Geometry check sheet. Reference: the model listing, model coordinates, mm. Face numbers are marked on the shaded views. A direction names the side the tool comes from. Give positions to 0.01 mm unless a question says otherwise; leave off trailing zeros. One line per question, with ' | ' between items. Start each with the question number.
Q1. Thickness scan on L1, parallel to Z at x = -89.5, y = -76; L2, parallel to Y at x = 70, z = 10.8; L3, parallel to Z at x = -86, y = -62. Record the ranges inside material, lowest first. Write a range as [from, to].
Q2. Set-up check for the marked faces 1 and 2: record each of +Z, -Z, +X, -X, +Y, -Y from which the full face is reachable in a straight line by a thin tool's end or side.
Q3. Section check A-A on z = 16.5. Count the separate pieces of the cut face and the enclosed holes in it, and give its area (3 significant figures).
Q4. Gauge pin test, flat ends, axial feed: P1, Ø5, axis at x = -50.5, y = 0, coming from the -Z side; P2, Ø2, axis at x = 66, z = 16.5, coming from the -Y side; P3, Ø4, axis at x = -24, z = 17, coming from the +Y side. Record the tip position at first contact, or that the pin passes through.
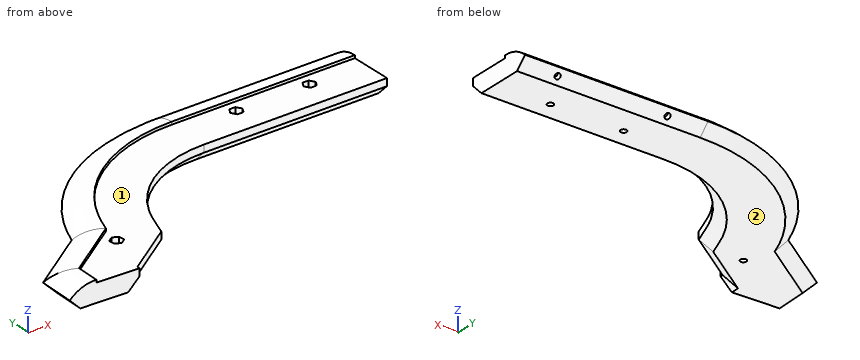
Autodesk Inventor part; units mm, degrees
ref_plane "Work Plane1" through (50, 0, 0) normal (-1, 0, 0) x (0, 0, 1)
ref_plane "Work Plane2" through (0, 14.1421, 14.1421) normal (0, 0, 1) x (1, 0, 0)
ref_plane "YZ Plane" through (0, 0, 0) normal (1, 0, 0) x (0, 1, 0)
sketch "Sketch1" plane through (0, 0, 0) normal (1, 0, 0) x (0, 1, 0)
  circle A0 centre (0, 0) radius 20
  line L0 (8.5, 8.5) -> (-16.9, 8.5)
  line L1 (8.5, 8.5) -> (8.5, -16.9)
  line L2 (0, 0) -> (0, 20)
  line L3 (0, 20) -> (-60.9241, 20)
  line L4 (-60.9241, 20) -> (-60.9241, 18.5)
  line L5 (-60.9241, 18.5) -> (0, 18.5)
  line L6 (0, 18.5) -> (0, 20)
  line L7 (0, 0) -> (14.1421, 14.1421)
  line L8 (0, 0) -> (20, 0)
  line L9 (-16.9, 8.5) -> (-16.9, 18.5)
  line L10 (-16.9, 8.5) -> (-22.9, 14.5)
  line L11 (-22.9, 14.5) -> (-22.9, 18.5)
  line L12 (12.3744, 12.3744) -> (12.1502, 13.2109)
  line L13 (11.3137, 13.435) -> (9.2071, 11.3284)
  line L14 (9.4313, 10.4919) -> (10.2678, 10.2678)
  line L15 (8.5, 8.5) -> (8.5, -16.9)
  line L16 (20, 0) -> (20, -60.9241)
  line L17 (20, -60.9241) -> (18.5, -60.9241)
  line L18 (18.5, -60.9241) -> (18.5, 0)
  line L19 (8.5, -16.9) -> (18.5, -16.9)
  line L20 (8.5, -16.9) -> (14.5, -22.9)
  line L21 (14.5, -22.9) -> (18.5, -22.9)
  arc A1 (9.2071, 11.3284) -> (9.4313, 10.4919) centre (9.5607, 10.9749) ccw
  arc A2 (12.1502, 13.2109) -> (11.3137, 13.435) centre (11.6673, 13.0815) ccw
  line L22 (10.4311, 10.4311) -> (9.483, 10.6851)
  arc A3 (9.3485, 11.187) -> (9.483, 10.6851) centre (9.5607, 10.9749) ccw
  line L23 (9.3485, 11.187) -> (11.4551, 13.2936)
  arc A4 (11.957, 13.1591) -> (11.4551, 13.2936) centre (11.6673, 13.0815) ccw
  line L24 (11.957, 13.1591) -> (12.2111, 12.2111)
  point P0 (0, 8.5)
  point P1 (-17.7041, 9.3041)
  point P2 (-16.9, 10.6953)
  dimension "d0" = 40
  dimension "d1" = 25.4
  dimension "d2" = 1.5
  dimension "d4" = 45
  dimension "d6" = 45
  dimension "d7" = 4
  dimension "d8" = 10
  dimension "d10" = 2.5
  dimension "d11" = 2.5
  dimension "d12" = 60
  dimension "d13" = 1.5
  dimension "d15" = 0.5
  dimension "d16" = 0.2
extrude "Extrusion1" add sketch "Sketch1" along normal blind 100 contours L7 L12 A2 L13 A1 L14 L0 L2 A0 | L7 L24 A4 L23 A3 L22 L14 A1 L13 A2 L12 | L5 L2 L0 L9 A0 | A0 L9 L5 | L7 L22 A3 L23 A4 L24 | L9 L10 A0 | A0 L10 L11 L5 L9
sketch "Sketch2" plane through (0, -22.9, 18.5) normal (0, 0, 1) x (1, 0, 0)
  line L0 (0, 22.9) -> (0, 0)
  line L1 (0, 0) -> (100, 0)
  line L2 (100, 22.9) -> (100, 0)
  line L3 (0, 22.9) -> (100, 22.9)
  line L4 (28.3257, 13.1) -> (26.6514, 16)
  line L5 (26.6514, 16) -> (28.3257, 18.9)
  line L6 (28.3257, 18.9) -> (31.6743, 18.9)
  line L7 (31.6743, 18.9) -> (33.3486, 16)
  line L8 (33.3486, 16) -> (31.6743, 13.1)
  line L9 (31.6743, 13.1) -> (28.3257, 13.1)
  line L10 (0, 6) -> (100, 6)
  circle A0 centre (30, 16) radius 1.65
  dimension "d20" = 10
  dimension "d21" = 5.8
  dimension "d22" = 30
  dimension "d25" = 3.3
extrude "Extrusion2" cut sketch "Sketch2" against normal blind 6 contours L4 L5 L6 L7 L8 L9 | A0
extrude "Extrusion3" cut sketch "Sketch2" against normal through all contours A0
sketch "Sketch3" plane through (0, -22.9, 18.5) normal (0, 0, 1) x (1, 0, 0)
  line L0 (0, 37.0421) -> (100, 37.0421)
  line L1 (0, 0) -> (100, 0)
  line L2 (0, 22.9) -> (0, 0)
  line L3 (0, 22.9) -> (0, 37.0421)
  line L4 (2.4384, 37.0421) -> (17.8575, 0)
  line L5 (0, 0) -> (100, 0)
  line L6 (2.4384, 37.0421) -> (0, 42.9)
  point P0 (0, 26.9698)
  dimension "d28" = 112.6
sketch "Sketch4" plane through (100, 14.1421, 14.1421) normal (0, 0.7071, -0.7071) x (-1, 0, 0)
  line L0 (100, 0) -> (0, 0)
  line L1 (0, -7.9792) -> (0, 0)
  line L2 (100, -7.9792) -> (0, -7.9792)
  circle A0 centre (80, -4) radius 1.5
  line L3 (100, -7.9792) -> (100, 0)
  line L4 (50, -7.9792) -> (50, 0)
  ellipse E0 centre (70, -18.8686) end of major axis (68.35, -18.8686) minor radius 1.1667
  point P0 (100, -20)
  dimension "d34" = 3
  dimension "d35" = 4
  dimension "d46" = 20
extrude "Extrusion5" cut sketch "Sketch4" against normal blind 3 contours A0
ref_plane "Work Plane1" through (50, 0, 0) normal (-1, 0, 0) x (0, 0, 1)
mirror "Mirror1" about plane through (50, 0, 0) normal (-1, 0, 0) of "Extrusion5", "Extrusion2", "Extrusion3"
ref_plane "Work Plane2" through (0, 14.1421, 14.1421) normal (0, 0, 1) x (1, 0, 0)
sketch "Sketch9" plane through (0, 14.1421, 14.1421) normal (0, 0, 1) x (1, 0, 0)
  line L0 (0, 0) -> (100, 0)
  line L1 (0, 0) -> (-127.2781, -88.4606) construction
  line L2 (0, -14.1421) -> (0, 0)
  arc A0 (0, 0) -> (-93.7282, -65.1428) centre (0, -100) ccw
  line L3 (-127.2781, -88.4606) -> (-93.7282, -65.1428)
  line L4 (-127.2781, -88.4606) -> (-128.0459, -108.4459)
  dimension "d61" = 155
  dimension "d62" = 145.2
  dimension "d63" = 100
  dimension "d66" = 127
  dimension "d67" = 20
sketch "Sketch10" plane through (0, 0, 0) normal (-1, 0, 0) x (0, 0, 1)
  line L0 (14.5, -22.9) -> (8.5, -16.9)
  line L1 (18.5, -22.9) -> (14.5, -22.9)
  line L2 (18.5, 0) -> (18.5, -22.9)
  line L3 (20, 0) -> (18.5, 0)
  arc A0 (20, 0) -> (14.1421, 14.1421) centre (0, 0) ccw
  line L4 (8.5, 8.5) -> (14.1421, 14.1421)
  line L5 (8.5, -16.9) -> (8.5, 8.5)
sweep "Sweep2" add profiles "Sketch10" path "Sketch9" path curves A0 L3 L4
sketch "Sketch11" plane through (100, -22.9, 18.5) normal (0, 0, 1) x (1, 0, 0)
  line L0 (-33.3486, 16) -> (-31.6743, 18.9)
  line L1 (-31.6743, 18.9) -> (-28.3257, 18.9)
  line L2 (-28.3257, 18.9) -> (-26.6514, 16)
  line L3 (-26.6514, 16) -> (-28.3257, 13.1)
  line L4 (-28.3257, 13.1) -> (-31.6743, 13.1)
  line L5 (-31.6743, 13.1) -> (-33.3486, 16)
  line L6 (-68.3257, 18.9) -> (-66.6514, 16)
  line L7 (-66.6514, 16) -> (-68.3257, 13.1)
  line L8 (-68.3257, 13.1) -> (-71.6743, 13.1)
  line L9 (-71.6743, 13.1) -> (-73.3486, 16)
  line L10 (-73.3486, 16) -> (-71.6743, 18.9)
  line L11 (-71.6743, 18.9) -> (-68.3257, 18.9)
  line L12 (-100, 0) -> (0, 0)
  line L13 (-100, 22.9) -> (0, 22.9)
  arc A0 (-100, 22.9) -> (-180.473, -33.0302) centre (-100, -62.9579) ccw
  line L14 (-180.473, -33.0302) -> (-182.0179, -37.1841)
  line L15 (-182.0179, -37.1841) -> (-213.4171, -59.0072)
  line L16 (-213.4171, -59.0072) -> (-213.9142, -71.9466)
  line L17 (-190.9723, -71.2953) -> (-191.0311, -72.8257)
  line L18 (-163.0556, -51.8928) -> (-190.9723, -71.2953)
  line L19 (-159.0093, -41.0125) -> (-163.0556, -51.8928)
  arc A1 (-100, 0) -> (-159.0093, -41.0125) centre (-100, -62.9579) ccw
  circle A2 centre (-30, 16) radius 1.65
  circle A3 centre (-70, 16) radius 1.65
  line L20 (-100, 31.4) -> (0, 31.4)
  line L21 (-100, 6) -> (0, 6)
  arc A4 (-100, 6) -> (-164.633, -38.9211) centre (-100, -62.9579) ccw
  line L22 (-164.633, -38.9211) -> (-168.0239, -48.039)
  line L23 (-168.0239, -48.039) -> (-196.853, -68.0757)
  line L24 (-196.853, -68.0757) -> (-197.0266, -72.5954)
  line L25 (-221.7481, -54.446) -> (-222.4079, -71.6203)
  line L26 (-189.0563, -31.7246) -> (-221.7481, -54.446)
  line L27 (-188.4399, -30.0674) -> (-189.0563, -31.7246)
  arc A5 (-100, 31.4) -> (-188.4399, -30.0674) centre (-100, -62.9579) ccw
  line L28 (-207.0193, -72.2115) -> (-206.6542, -62.7097)
  line L29 (-206.6542, -62.7097) -> (-176.3043, -41.616)
  line L30 (-176.3043, -41.616) -> (-174.0058, -35.4354)
  arc A6 (-100, 16) -> (-174.0058, -35.4354) centre (-100, -62.9579) ccw
  line L31 (-100, 16) -> (0, 16)
  line L32 (-186.0175, -48.3668) -> (-186.2977, -45.0299)
  line L33 (-186.2977, -45.0299) -> (-183.548, -43.1188)
  line L34 (-183.548, -43.1188) -> (-180.5181, -44.5446)
  line L35 (-180.5181, -44.5446) -> (-180.2379, -47.8815)
  line L36 (-180.2379, -47.8815) -> (-182.9876, -49.7926)
  line L37 (-182.9876, -49.7926) -> (-186.0175, -48.3668)
  circle A7 centre (-183.2678, -46.4557) radius 1.65
  point P0 (-181.6127, -48.8371)
  point P1 (-191.4793, -52.1629)
  dimension "d68" = 10
  dimension "d70" = 5.8
  dimension "d75" = 3.3
  dimension "d76" = 10
extrude "Extrusion7" cut sketch "Sketch11" against normal through all contours A7 L29 | L29 A7
extrude "Extrusion8" cut sketch "Sketch11" against normal blind 6 contours L35 L36 L37 L29 A7 | L29 A7 L32 L33 L34 | A7 L29 | L29 A7
sketch "Sketch12" plane through (100, -22.9, 18.5) normal (0, 0, 1) x (1, 0, 0)
  line L0 (-186.0175, -48.3668) -> (-186.2977, -45.0299)
  line L1 (-186.2977, -45.0299) -> (-183.548, -43.1188)
  line L2 (-183.548, -43.1188) -> (-180.5181, -44.5446)
  line L3 (-180.5181, -44.5446) -> (-180.2379, -47.8815)
  line L4 (-180.2379, -47.8815) -> (-182.9876, -49.7926)
  line L5 (-182.9876, -49.7926) -> (-186.0175, -48.3668)
  line L6 (-33.3486, 16) -> (-31.6743, 18.9)
  line L7 (-31.6743, 18.9) -> (-28.3257, 18.9)
  line L8 (-28.3257, 18.9) -> (-26.6514, 16)
  line L9 (-26.6514, 16) -> (-28.3257, 13.1)
  line L10 (-28.3257, 13.1) -> (-31.6743, 13.1)
  line L11 (-31.6743, 13.1) -> (-33.3486, 16)
  line L12 (-68.3257, 18.9) -> (-66.6514, 16)
  line L13 (-66.6514, 16) -> (-68.3257, 13.1)
  line L14 (-68.3257, 13.1) -> (-71.6743, 13.1)
  line L15 (-71.6743, 13.1) -> (-73.3486, 16)
  line L16 (-73.3486, 16) -> (-71.6743, 18.9)
  line L17 (-71.6743, 18.9) -> (-68.3257, 18.9)
  line L18 (-100, 0) -> (0, 0)
  line L19 (0, 22.9) -> (0, 0)
  line L20 (-100, 22.9) -> (0, 22.9)
  arc A0 (-100, 22.9) -> (-180.473, -33.0302) centre (-100, -62.9579) ccw
  line L21 (-180.473, -33.0302) -> (-182.0179, -37.1841)
  line L22 (-182.0179, -37.1841) -> (-213.4171, -59.0072)
  line L23 (-213.4171, -59.0072) -> (-213.9142, -71.9466)
  line L24 (-191.0311, -72.8257) -> (-213.9142, -71.9466)
  line L25 (-190.9723, -71.2953) -> (-191.0311, -72.8257)
  line L26 (-163.0556, -51.8928) -> (-190.9723, -71.2953)
  line L27 (-159.0093, -41.0125) -> (-163.0556, -51.8928)
  arc A1 (-100, 0) -> (-159.0093, -41.0125) centre (-100, -62.9579) ccw
properties part number "ESQUINA_REDONDEADA_R20" material "Steel, Mild, Welded"
Working result:
1) L1: z = [8.5, 18.5] | L2: y = [-19.2, -8.55], [-5.25, 10.8] | L3: z = [8.5, 19.99]
2) face 1: +Z, +X, -Y | face 2: -Z, +X, -X, +Y, -Y
3) separate pieces: 1 | enclosed holes: 3 | area: 8,490 mm2
4) P1: stops at z = 11.25 | P2: stops at y = -22.9 | P3: stops at y = 10.33
